Read the model definition and answer for the solid it produces. Units are mm, in the model's axes. A direction names the side the tool comes from. Give positions to 0.01 mm unless a question says otherwise; leave off trailing zeros. Loops run counter-clockwise (first coordinate to the right, second up) from the corner with the lowest first, then second, coordinate; pieces in that order, holes last. Notation, with made-up numbers: (80, -8) -> (128, -8) arc R26 cw to (128, 31) -> close; hole circle Ø3 at (-33, 58). An arc over 180 degrees is marked (long way). Return JSON: item names as keys, results as strings. Group by question number.
from build123d import *

# Parameters (mm, degrees)
SKETCH1_W         = 52
SKETCH1_H         = 38
SKETCH1_R         = 1.5
SKETCH1_R_2       = 9.55
FACE_IN_DEPTH     = 5
SKETCH8_W         = 8
SKETCH8_H         = 38
BOTTOM_DEPTH      = 38
FILLET1_R         = 5
SKETCH10_W        = 52
SKETCH10_H        = 38
FACE_OUT_DEPTH    = 3
SKETCH12_R        = 2.5
SCREW_HOLES_DEPTH = 8


with BuildPart() as part:
    # Sketch1 → Face_In (new body)
    with BuildSketch(Plane.XY):
        with Locations((26, 19)):
            Rectangle(SKETCH1_W, SKETCH1_H)
        with Locations((43.192388155, 28.192388155)):
            Circle(SKETCH1_R, mode=Mode.SUBTRACT)
        with Locations((43.192388155, 9.807611845)):
            Circle(SKETCH1_R, mode=Mode.SUBTRACT)
        with Locations((24.807611845, 9.807611845)):
            Circle(SKETCH1_R, mode=Mode.SUBTRACT)
        with Locations((24.807611845, 28.192388155)):
            Circle(SKETCH1_R, mode=Mode.SUBTRACT)
        with Locations((34, 19)):
            Circle(SKETCH1_R_2, mode=Mode.SUBTRACT)
    extrude(amount=FACE_IN_DEPTH)

    # Sketch8 → Bottom (add)
    with BuildSketch(Plane(origin=(0, 0, 0), x_dir=(-1, 0, 0), z_dir=(0, 0, -1))):
        with Locations((-4, 19)):
            Rectangle(SKETCH8_W, SKETCH8_H)
    extrude(amount=BOTTOM_DEPTH)

    # Fillet1
    fillet1_edges = [part.edges().sort_by_distance(p)[0] for p in [
        (8, 19, 0),
    ]]
    fillet(fillet1_edges, radius=FILLET1_R)

    # Sketch10 → Face_Out (add)
    with BuildSketch(Plane.XY.offset(5)):
        with Locations((26, 19)):
            Rectangle(SKETCH10_W, SKETCH10_H)
        with BuildLine():
            ThreePointArc((42.621806472, 24.992866856), (45.490485194, 30.490485194), (39.992866856, 27.621806472))
            ThreePointArc((39.992866856, 27.621806472), (34, 29.5), (28.007133144, 27.621806472))
            ThreePointArc((28.007133144, 27.621806472), (22.509514806, 30.490485194), (25.378193528, 24.992866856))
            ThreePointArc((25.378193528, 24.992866856), (23.5, 19), (25.378193528, 13.007133144))
            ThreePointArc((25.378193528, 13.007133144), (22.509514806, 7.509514806), (28.007133144, 10.378193528))
            ThreePointArc((28.007133144, 10.378193528), (34, 8.5), (39.992866856, 10.378193528))
            ThreePointArc((39.992866856, 10.378193528), (45.490485194, 7.509514806), (42.621806472, 13.007133144))
            ThreePointArc((42.621806472, 13.007133144), (44.5, 19), (42.621806472, 24.992866856))
        make_face(mode=Mode.SUBTRACT)
    extrude(amount=FACE_OUT_DEPTH)

    # Sketch12 → Screw Holes (cut)
    with BuildSketch(Plane.ZY):
        with Locations((-8, 30)):
            Circle(SKETCH12_R)
        with Locations((-30, 30)):
            Circle(SKETCH12_R)
        with Locations((-8, 8)):
            Circle(SKETCH12_R)
        with Locations((-30, 8)):
            Circle(SKETCH12_R)
    extrude(amount=-SCREW_HOLES_DEPTH, mode=Mode.SUBTRACT)


solid = part.part
1. Section B-B on x = 34 is taken. Determine the outline of the cut face in (y, z).
2. Section D-D on y = 23 is taken. Determine the outline of the cut face in (x, z).
3. Flat-ended cylindrical pins translate along their axes: pin 1 Ø7.5 at (x, y) = (40, 19.5) entering from +Z; pin 2 Ø6 at (y, z) = (14, -21) entering from +X; pin 3 Ø3.5 at (x, y) = (24.81, 9.81) entering from -Z. Find the tip coordinate at first contact, or state that the pin passes through.
4. Straight lines are drawn through the part: line 1 (Y direction, x = 34, z = 3.15); line 2 (Y direction, x = 2, z = -8); line 3 (Z direction, x = 18, y = 2.5). For each, find the intervals that lie inside material, in ascending order. Write a range as from..to.
5. Determine the mould class of faces 3 (the cylindrical face through (44.58, 27.62, 2.46)), 4 (the flat face through (0, 19, -15)), 5 (the flat face through (8, 19, -21)), 6 (the cylindrical face through (3.94, 31.69, -31.84)) for opening direction X: pulls with the +X half, pulls with the -X half, needs draft (parallel to the pull), parting line crosses it, or undercut.
6. Which of the six approach directions +Z, -Z, +X, -X, +Y, -Y give full straight-line access (tool end or side, diameter ignored) to faces 1 (the cylindrical face through (44.578, 9.233, 2.465)), 2 (the cylindrical face through (33.9, 8.5, 6.5))?
7. Section A-A on y = 19 is taken. Determine the outline of the cut face in (x, z), then the cut area to 3 significant figures.
8. Section C-C on z = -8 is taken. Determine the outline of the cut face in (x, y), then the cut area to 3 significant figures.
Completed:
{
 "1": {"outline": "(0, 0) -> (9.45, 0) -> (9.45, 5) -> (8.5, 5) -> (8.5, 8) -> (0, 8) -> close; (28.55, 0) -> (38, 0) -> (38, 8) -> (29.5, 8) -> (29.5, 5) -> (28.55, 5) -> close"},
 "2": {"outline": "(0, -38) -> (8, -38) -> (8, -5) arc R5 cw to (13, 0) -> (25.33, 0) -> (25.33, 5) -> (24.29, 5) -> (24.29, 8) -> (0, 8) -> close; (42.67, 0) -> (52, 0) -> (52, 8) -> (43.71, 8) -> (43.71, 5) -> (42.67, 5) -> close"},
 "3": {"pin 1": "stops at z = 5", "pin 2": "stops at x = 8", "pin 3": "stops at z = 0"},
 "4": {"line 1": "y = 0..9.45, 28.55..38", "line 2": "y = 0..5.5, 10.5..27.5, 32.5..38", "line 3": "z = 0..8"},
 "5": {"face 3": "undercut", "face 4": "pulls with the -X half", "face 5": "pulls with the +X half", "face 6": "needs draft"},
 "6": {"face 1": "+Z, -Z", "face 2": "+Z"},
 "7": {"outline": "(0, -38) -> (8, -38) -> (8, -5) arc R5 cw to (13, 0) -> (24.45, 0) -> (24.45, 5) -> (23.5, 5) -> (23.5, 8) -> (0, 8) -> close; (43.55, 0) -> (52, 0) -> (52, 8) -> (44.5, 8) -> (44.5, 5) -> (43.55, 5) -> close", "area": "567 mm²"},
 "8": {"outline": "(0, 0) -> (8, 0) -> (8, 5.5) -> (0, 5.5) -> close; (0, 10.5) -> (8, 10.5) -> (8, 27.5) -> (0, 27.5) -> close; (0, 32.5) -> (8, 32.5) -> (8, 38) -> (0, 38) -> close", "area": "224 mm²"}
}
